Build history of the part. All positions in model axes, mm. A direction names the side the tool comes from. Round coordinates to 2 decimals unless told otherwise and drop trailing zeros. Loops run counter-clockwise (first coordinate to the right, second up) from the corner with the lowest first, then second, coordinate; pieces in that order, holes last. Notation, with made-up numbers: (-33, 68.25) - (11, 68.25) arc R29 cw to (11, 95.25) - close; hole circle Ø3 at (38, 34.25). An arc over 180 degrees is marked (long way). Use one line per item in the form item = value. Start each with the question number.
Q1. Saw through at A-A (x = 0). Give the cut face in (y, z) (3 decimals).
Q2. Saw through at B-B (z = 42.5). Give the cut face in (x, y).
Q3. Saw through at D-D (z = 12.25). Give the cut face in (x, y) (3 decimals), then the cut area to 3 significant figures.
Q4. Drill centre lines: line 1 (Z direction, x = 5, y = 1.1); line 2 (X direction, y = 4, z = 11); line 3 (X direction, y = 0.45, z = 12.25) (3 decimals). Where is each one in solid material? Low to high.
Q5. Mould opens along Z. For faces 1 (the face through (14.37, 5, 22)), 2 (the face through (-2, 1, 0)), 3 (the face through (13.57, 11.14, 2.1)), 4 (the face through (-0.853, 0.799, 36.091)) say: released by +Z, released by -Z, zero draft, split by the parting line, or undercut.
Q6. Saw through at C-C (y = 7.5). Give the cut face in (x, z).
Q7. Pin check, flat tips, straight feed: pin 1 (1.5 mm diameter, centred on x = 4, z = 31, fed in from +Y); pin 2 (1.8 mm diameter, centred on x = 5, z = 27.25, fed in from +Y); pin 3 (1.3 mm diameter, centred on x = 14, z = 30, fed in from +Y). Stop position of each tip, or through.
Q8. 3-axis set-ups, long thin cutter, end or side, ignore diameter. For faces 5 (the face through (-13.57, 11.14, 2.1)), 6 (the face through (-2, 1, 44.5)): which of +Z, -Z, +X, -X, +Y, -Y reach the whole face in a straight line?
```python
from build123d import *

# Parameters (mm, degrees)
BOSS_EXTRUDE1_DEPTH = 44.5
SKETCH2_R           = 0.5
CUT_EXTRUDE1_DEPTH  = 44.5
SKETCH3_R           = 3.935
SKETCH3_R_2         = 1
CUT_EXTRUDE2_DEPTH  = 20.5


with BuildPart() as part:
    # Sketch1 → Boss-Extrude1 (new body)
    with BuildSketch(Plane.XY):
        Polygon((0, 0), (-14.37, 0), (-14.37, 12), (-12.75, 12), (-12.75, 1.62), (0, 1.62), align=None)
    boss_extrude1 = extrude(amount=BOSS_EXTRUDE1_DEPTH)

    # Sketch2 → Cut-Extrude1 (cut)
    with BuildSketch(Plane.ZY.offset(14.37)):
        with Locations((2, 9)):
            Circle(SKETCH2_R)
        with Locations((42.5, 9)):
            Circle(SKETCH2_R)
        with BuildLine():
            Line((3, 9), (41.5, 9))
            ThreePointArc((41.5, 9), (42.378679656, 11.121320344), (44.5, 12))
            Line((44.5, 12), (44.5, 14.744822673))
            Line((44.5, 14.744822673), (0, 14.744822673))
            Line((0, 14.744822673), (0, 12))
            ThreePointArc((0, 12), (2.121320344, 11.121320344), (3, 9))
        make_face()
    cut_extrude1 = extrude(amount=-CUT_EXTRUDE1_DEPTH, mode=Mode.SUBTRACT)

    # Mirror1: Boss-Extrude1, Cut-Extrude1 across plane
    add(boss_extrude1.mirror(Plane(origin=(0, 1.62, 44.5), x_dir=(0, 0, 1), z_dir=(-1, 0, 0))))
    add(cut_extrude1.mirror(Plane(origin=(0, 1.62, 44.5), x_dir=(0, 0, 1), z_dir=(-1, 0, 0))), mode=Mode.SUBTRACT)

    # Sketch3 → Cut-Extrude2 (cut)
    with BuildSketch(Plane(origin=(0, 0, 0), x_dir=(1, 0, 0), z_dir=(0, 1, 0))):
        with Locations((0, -12.25)):
            Circle(SKETCH3_R)
        with Locations((-5, -7.25)):
            Circle(SKETCH3_R_2)
        with Locations((5, -7.25)):
            Circle(SKETCH3_R_2)
        with Locations((5, -17.25)):
            Circle(SKETCH3_R_2)
        with Locations((-5, -17.25)):
            Circle(SKETCH3_R_2)
        with Locations((0, -22.25)):
            Circle(SKETCH3_R)
        with Locations((-5, -27.25)):
            Circle(SKETCH3_R_2)
        with Locations((5, -27.25)):
            Circle(SKETCH3_R_2)
        with Locations((0, -32.25)):
            Circle(SKETCH3_R)
        with Locations((-5, -37.25)):
            Circle(SKETCH3_R_2)
        with Locations((5, -37.25)):
            Circle(SKETCH3_R_2)
    extrude(amount=CUT_EXTRUDE2_DEPTH, mode=Mode.SUBTRACT)


solid = part.part
```
Report:
q1.outline = (0, 0) - (1.62, 0) - (1.62, 8.315) - (0, 8.315) - close; (0, 16.185) - (1.62, 16.185) - (1.62, 18.315) - (0, 18.315) - close; (0, 26.185) - (1.62, 26.185) - (1.62, 28.315) - (0, 28.315) - close; (0, 36.185) - (1.62, 36.185) - (1.62, 44.5) - (0, 44.5) - close
q2.outline = (-14.37, 0) - (14.37, 0) - (14.37, 8.5) - (12.75, 8.5) - (12.75, 1.62) - (-12.75, 1.62) - (-12.75, 8.5) - (-14.37, 8.5) - close; (-14.37, 9.5) - (-12.75, 9.5) - (-12.75, 11.24) - (-14.37, 11.24) - close; (12.75, 9.5) - (14.37, 9.5) - (14.37, 11.24) - (12.75, 11.24) - close
q3.outline = (-14.37, 0) - (-3.935, 0) - (-3.935, 1.62) - (-12.75, 1.62) - (-12.75, 9) - (-14.37, 9) - close; (3.935, 0) - (14.37, 0) - (14.37, 9) - (12.75, 9) - (12.75, 1.62) - (3.935, 1.62) - close
q3.area = 57.7 mm²
q4.line_1 = 0 to 6.25, 8.25 to 16.25, 18.25 to 26.25, 28.25 to 36.25, 38.25 to 44.5
q4.line_2 = -14.37 to -12.75, 12.75 to 14.37
q4.line_3 = -14.37 to -3.935, 3.935 to 14.37
q5.face_1 = zero draft
q5.face_2 = released by -Z
q5.face_3 = undercut
q5.face_4 = undercut
q6.outline = (-14.37, 0) - (-12.75, 0) - (-12.75, 44.5) - (-14.37, 44.5) - close; (12.75, 0) - (14.37, 0) - (14.37, 44.5) - (12.75, 44.5) - close
q7.pin_1 = 1.62
q7.pin_2 = through
q7.pin_3 = 9
q8.face_5 = +X, -X, +Y
q8.face_6 = +Z, +X, -X, +Y, -Y
